Design review of the part built by this model. Coordinates are the model's own, in mm. A direction names the side the tool comes from. Coordinates: 2 decimals unless noted, no trailing zeros. Write each loop counter-clockwise with the first axis right and the second up, starting at its lowest first coordinate (ties: lowest second). Pieces come first, ordered by that corner, then holes.
```python
from build123d import *

# Parameters (mm, degrees)
F0_R     = 1.25
F1_DEPTH = 1


with BuildPart() as f1:
    # F0 (on Top) → F1 (new body)
    with BuildSketch(Plane.XY):
        Polygon((15.25, 9.5), (15.25, 14.25), (-15.25, 14.25), (-15.25, 9.5), (-15.25, -9.5), (-15.25, -14.25), (15.25, -14.25), (15.25, -9.5), align=None)
        with BuildLine():
            Line((-15.25, -9.5), (-15.25, 9.5))
            Line((-15.25, 9.5), (-20.541877, 1.519803))
            ThreePointArc((-20.541877, 1.519803), (-21, 0), (-20.541877, -1.519803))
            Line((-20.541877, -1.519803), (-15.25, -9.5))
        make_face()
        with Locations((-18.25, 0)):
            Circle(F0_R, mode=Mode.SUBTRACT)
        with BuildLine():
            Line((20.541877, 1.519803), (15.25, 9.5))
            Line((15.25, 9.5), (15.25, -9.5))
            Line((15.25, -9.5), (20.541877, -1.519803))
            ThreePointArc((20.541877, -1.519803), (21, 0), (20.541877, 1.519803))
        make_face()
        with Locations((18.25, 0)):
            Circle(F0_R, mode=Mode.SUBTRACT)
    extrude(amount=F1_DEPTH)


solid = f1.part
```
(1) Consider section A-A (y = 0). Give the boundary of the cut face in (x, z).
(2) Consider section B-B (x = -18.25). Give the boundary of the cut face in (y, z), plus the area to 3 significant figures.
(3) Consider section D-D (y = -11.5). Give the boundary of the cut face in (x, z).
(4) Wall thickness on line 1 (Y direction, x = -19, z = 0.55); line 2 (Y direction, x = -18.25, z = 0.7); line 3 (Y direction, x = 16, z = 0.9): over which ranges is each line inside the solid? List them lowest first.
(5) Mouldability with a two-part tool opening along Y and no side actions: class faces 6 (the cylindrical face through (-17.095, -0.479, 0.493)), 7 (the flat face through (-0.2, -14.25, 0.5)), 8 (the flat face through (15.25, 11.8, 0.5)) as +Y half, -Y half, draft (parallel to the pull), parting line (faces both ways), or undercut.
(6) Insertion check: pin 1 Ø0.5 at (y, z) = (-12.5, 0.5) entering from +X; pin 2 Ø1.5 at (x, y) = (-18.25, 0) entering from -Z. Each pin has a flat end and moves straight along its axis. Give the tip position at first contact, or say it passes through.
(7) For faces 1 (the flat face through (-15.25, 11.9, 0.5)), 2 (the flat face through (-15.25, -11.8, 0.5)), 3 (the flat face through (15.25, -11.9, 0.5)), 4 (the flat face through (0, 0, 1)), 5 (the flat face through (0, 0, 0)), list the 3-axis set-ups (+Z, -Z, +X, -X, +Y, -Y) from which the entire face can be reached by the end or side of a thin tool; tool diameter is ignored.
(8) Consider section C-C (z = 0.2). Give the boundary of the cut face in (x, y).
Results:
1. outline: (-21, 0) - (-19.5, 0) - (-19.5, 1) - (-21, 1) - close; (-17, 0) - (17, 0) - (17, 1) - (-17, 1) - close; (19.5, 0) - (21, 0) - (21, 1) - (19.5, 1) - close
2. outline: (-4.98, 0) - (-1.25, 0) - (-1.25, 1) - (-4.98, 1) - close; (1.25, 0) - (4.98, 0) - (4.98, 1) - (1.25, 1) - close
2. area: 7.45 mm2
3. outline: (-15.25, 0) - (15.25, 0) - (15.25, 1) - (-15.25, 1) - close
4. line 1: y = -3.84 to -1, 1 to 3.84
4. line 2: y = -4.98 to -1.25, 1.25 to 4.98
4. line 3: y = -8.37 to 8.37
5. face 6: undercut
5. face 7: -Y half
5. face 8: draft
6. pin 1: stops at x = 15.25
6. pin 2: passes through
7. face 1: +Z, -Z, -X, +Y
7. face 2: +Z, -Z, -X, -Y
7. face 3: +Z, -Z, +X, -Y
7. face 4: +Z, +X, -X, +Y, -Y
7. face 5: -Z, +X, -X, +Y, -Y
8. outline: (-20.54, -1.52) - (-15.25, -9.5) - (-15.25, -14.25) - (15.25, -14.25) - (15.25, -9.5) - (20.54, -1.52) arc R2.75 ccw to (20.54, 1.52) - (15.25, 9.5) - (15.25, 14.25) - (-15.25, 14.25) - (-15.25, 9.5) - (-20.54, 1.52) arc R2.75 ccw to start; hole circle Ø2.5 at (-18.25, 0); hole circle Ø2.5 at (18.25, 0)
